Geometry: final body of the model. Coordinates: model frame, mm. Give positions to 0.01 mm unless a question says otherwise; leave off trailing zeros. Order: outer loops, then holes, each group sorted by start corner. A loop starts at its lowest first (then second) coordinate and runs counter-clockwise, first axis right, second up. Notation, with made-up numbers: M -9,-28 L 25,-28 A24 cw 25,7 Z; hole C 76.5,25 d6. An arc over 180 degrees is marked long. One line per item, written item: value. Start each with the question number.
```python
from build123d import *

# Parameters (mm, degrees)
BOSS_EXTRUDE1_DEPTH                                 = 6
CSK_FOR_M3_COUNTERSUNK_FLAT_HEAD_SCREW1_D           = 3.2
CSK_FOR_M3_COUNTERSUNK_FLAT_HEAD_SCREW1_CSINK_D     = 7.3
CSK_FOR_M3_COUNTERSUNK_FLAT_HEAD_SCREW1_CSINK_ANGLE = 90


with BuildPart() as part:
    # Sketch1 → Boss-Extrude1 (new body)
    with BuildSketch(Plane.XY):
        Polygon((-40, 42.599696279), (-40, -75.400303721), (-39, -76.400303721), (23.564831516, -76.400303721), (60, -44.727694967), (60, 42.599696279), (59, 43.599696279), (-39, 43.599696279), align=None)
    extrude(amount=BOSS_EXTRUDE1_DEPTH)

    # CSK for M3 Countersunk Flat Head Screw1 (through all)
    with Locations(Plane(origin=(-34, 37.599696279, 6), x_dir=(1, 0, 0), z_dir=(0, 0, 1))):
        with Locations((0, 0), (88, 0), (88, -54), (0, -54), (0, -108), (55.321523439, -108)):
            CounterSinkHole(CSK_FOR_M3_COUNTERSUNK_FLAT_HEAD_SCREW1_D / 2, CSK_FOR_M3_COUNTERSUNK_FLAT_HEAD_SCREW1_CSINK_D / 2, counter_sink_angle=CSK_FOR_M3_COUNTERSUNK_FLAT_HEAD_SCREW1_CSINK_ANGLE)


solid = part.part
```
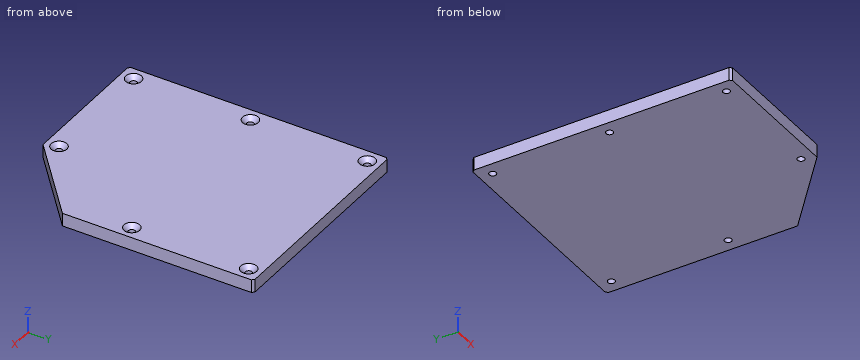
Q1. Section query A-A on x = -34. Return loops of the section in (y, z), and give its area (3 significant figures).
Q2. Section query C-C on z = 2.8. Return loops of the section in (x, y).
Q3. Section query D-D on y = -65. Return loops of the section in (x, z).
Q4. Ray query, line 1 along Y through (x, z) = (-34, 2); line 2 along Y through (x, z) = (54, 3.05); line 3 along X through (y, z) = (-64, 4.6). Return the intervals inside material, ascending. Write a range as [from, to].
Q5. Contact query for flat-ended pins moving along their axis: pin 1 (3.5 mm diameter, centred on x = -34, y = 37.6, fed in from +Z); pin 2 (3 mm diameter, centred on x = 21.32, y = -70.4, fed in from +Z); pin 3 (5 mm diameter, centred on x = -34, y = -16.4, fed in from +Z). Output: stop coordinate, or through.
Q6. Section query B-B on x = 54. Return loops of the section in (y, z).
Results below:
1. outline: M -76.4,0 L -72,0 L -72,3.95 L -74.05,6 L -76.4,6 Z; M -68.8,0 L -18,0 L -18,3.95 L -20.05,6 L -66.75,6 L -68.8,3.95 Z; M -14.8,0 L 36,0 L 36,3.95 L 33.95,6 L -12.75,6 L -14.8,3.95 Z; M 39.2,0 L 43.6,0 L 43.6,6 L 41.25,6 L 39.2,3.95 Z
1. area: 650 mm2
2. outline: M -40,-75.4 L -39,-76.4 L 23.56,-76.4 L 60,-44.73 L 60,42.6 L 59,43.6 L -39,43.6 L -40,42.6 Z; hole C -34,-70.4 d3.2; hole C -34,-16.4 d3.2; hole C -34,37.6 d3.2; hole C 21.32,-70.4 d3.2; hole C 54,-16.4 d3.2; hole C 54,37.6 d3.2
3. outline: M -40,0 L 36.68,0 L 36.68,6 L -40,6 Z
4. line 1: [-76.4, -72], [-68.8, -18], [-14.8, 36], [39.2, 43.6]
4. line 2: [-49.94, -18], [-14.8, 36], [39.2, 43.6]
4. line 3: [-40, 37.83]
5. pin 1: z = 4.1
5. pin 2: through
5. pin 3: z = 4.85
6. outline: M -49.94,0 L -18,0 L -18,3.95 L -20.05,6 L -49.94,6 Z; M -14.8,0 L 36,0 L 36,3.95 L 33.95,6 L -12.75,6 L -14.8,3.95 Z; M 39.2,0 L 43.6,0 L 43.6,6 L 41.25,6 L 39.2,3.95 Z
